from build123d import *

# Parameters (mm, degrees)
F1_DEPTH = 7
F3_DEPTH = 6
F4_W     = 2.3945512949
F4_H     = 2.3532351479
F5_DEPTH = 6


with BuildPart() as f1:
    # F0 (on Top) → F1 (new body)
    with BuildSketch(Plane.XY):
        Polygon((-10.1898079023, -17.6492650062), (10.1898079023, -17.6492650062), (20.3796158046, 0), (10.1898079023, 17.6492650062), (-10.1898079023, 17.6492650062), (-20.3796158046, 0), align=None)
    extrude(amount=F1_DEPTH)

    # F2 (on face) → F3 (cut)
    with BuildSketch(Plane.XY.offset(7)):
        Polygon((-8.8311669562, -15.2960298583), (8.8311669562, -15.2960298583), (17.6623339124, 0), (8.8311669562, 15.2960298583), (-8.8311669562, 15.2960298583), (-17.6623339124, 0), align=None)
    extrude(amount=-F3_DEPTH, mode=Mode.SUBTRACT)

    # F4 (on face) → F5 (cut)
    with BuildSketch(Plane.XY.offset(7)):
        with Locations((0.0150980777, -16.4726474322)):
            Rectangle(F4_W, F4_H)
    extrude(amount=-F5_DEPTH, mode=Mode.SUBTRACT)


solid = f1.part
The model under review builds one solid part; all positions refer to its coordinate system, in mm. A direction names the side the tool comes from. Coordinates: 2 decimals unless noted, no trailing zeros. Write each loop counter-clockwise with the first axis right and the second up, starting at its lowest first coordinate (ties: lowest second). Pieces come first, ordered by that corner, then holes. Notation, with made-up numbers: (76.25, 26) -> (101.25, 26) arc R10 ccw to (101.25, 44) -> close; hole circle Ø8 at (74, 40). An arc over 180 degrees is marked (long way). Answer in a Markdown table with one row per item.
1. For faces 4 (the flat face through (-13.18, 7.76, 4.04)), 5 (the flat face through (-15.213, 8.948, 3.451)), 6 (the flat face through (-1.182, -16, 4)), list the 3-axis set-ups (+Z, -Z, +X, -X, +Y, -Y) from which the entire face can be reached by the end or side of a thin tool; tool diameter is ignored.
Answers below:
| item | result |
|---|---|
| face 4 | +Z |
| face 5 | +Z, -Z, -X, +Y |
| face 6 | +Z, -Y |
2. Draft analysis for pull direction X (two halves, no side actions). For faces 1 (the flat face through (0, 15.296, 4)), 2 (the flat face through (15.213, -8.948, 3.451)), 3 (the flat face through (0, 17.649, 3)), state which applies: +X half, -X half, draft (parallel to the pull), parting line (faces both ways), or undercut.
Answers below:
| item | result |
|---|---|
| face 1 | undercut |
| face 2 | +X half |
| face 3 | draft |
3. We need section A-A, the plane z = 0.5. State the section outline as (x, y) points.
Answers below:
| item | result |
|---|---|
| outline | (-20.38, 0) -> (-10.19, -17.65) -> (10.19, -17.65) -> (20.38, 0) -> (10.19, 17.65) -> (-10.19, 17.65) -> close |
4. We need section C-C, the plane x = -15.5. State the section outline as (y, z) points.
Answers below:
| item | result |
|---|---|
| outline | (-8.45, 0) -> (8.45, 0) -> (8.45, 7) -> (3.75, 7) -> (3.75, 1) -> (-3.75, 1) -> (-3.75, 7) -> (-8.45, 7) -> close |
5. Clearance check with flat-ended pins moving along their axes: pin 1 Ø0.7 at (y, z) = (-16.5, 4) entering from -X; pin 2 Ø2 at (x, z) = (11, 6) entering from +Y; pin 3 Ø1.2 at (y, z) = (-17, 3.5) entering from +X; pin 4 Ø2 at (y, z) = (-4.5, 4.5) entering from -X. State where each tip first meets the part, or that it passes through.
Answers below:
| item | result |
|---|---|
| pin 1 | stops at x = -11.06 |
| pin 2 | stops at y = 17.65 |
| pin 3 | stops at x = 10.91 |
| pin 4 | stops at x = -18.36 |
6. We need section D-D, the plane z = 6.25. State the section outline as (x, y) points, and give its area (3 significant figures).
Answers below:
| item | result |
|---|---|
| outline | (-20.38, 0) -> (-10.19, -17.65) -> (-1.18, -17.65) -> (-1.18, -15.3) -> (-8.83, -15.3) -> (-17.66, 0) -> (-8.83, 15.3) -> (8.83, 15.3) -> (17.66, 0) -> (8.83, -15.3) -> (1.21, -15.3) -> (1.21, -17.65) -> (10.19, -17.65) -> (20.38, 0) -> (10.19, 17.65) -> (-10.19, 17.65) -> close |
| area | 263 mm^2 |
7. We need section B-B, the plane y = -10.5. State the section outline as (x, z) points.
Answers below:
| item | result |
|---|---|
| outline | (-14.32, 0) -> (14.32, 0) -> (14.32, 7) -> (11.6, 7) -> (11.6, 1) -> (-11.6, 1) -> (-11.6, 7) -> (-14.32, 7) -> close |
8. Wall thickness on probe 1 along Y at (x, z) = (-8.5, 5.25); probe 2 along Z at (x, y) = (-7, 12); probe 3 along X at (y, z) = (13.5, 3.75): over which ranges is each line inside the solid? List them lowest first. Write a range as [from, to].
Answers below:
| item | result |
|---|---|
| probe 1 | y = [-17.65, -15.3], [15.3, 17.65] |
| probe 2 | z = [0, 1] |
| probe 3 | x = [-12.59, -9.87], [9.87, 12.59] |
